Part model, mm, in its own coordinate system. Face numbers are marked on the shaded views. Round coordinates to 2 decimals unless told otherwise and drop trailing zeros. Write each loop counter-clockwise with the first axis right and the second up, starting at its lowest first coordinate (ties: lowest second). Pieces come first, ordered by that corner, then holes. Notation, with made-up numbers: M 69.25,71.25 L 89.25,71.25 A26 cw 89.25,95.25 Z; hole C 5.5,-18 d9. An arc over 180 degrees is marked long. Use one line per item in the form item = value. Start each with the question number.
Item 1: Mould opens along X. For the marked faces 1, 2 and 3 say: +X half, -X half, draft (parallel to the pull), parting line (faces both ways), or undercut.
Item 2: Cut at C-C, the plane x = 45. Give the cut face in (y, z), then the cut area to 3 significant figures.
Item 3: Probe L1, parallel to X at y = 12.25, z = 0; L2, parallel to Y at x = -36, z = 30.5; L3, parallel to X at y = 15.5, z = 0. List the from-to ranges inside material, lowest first.
Item 4: Cut at D-D, the plane y = 18.5. Give the cut face in (x, z), then the cut area to 3 significant figures.
Item 5: Flat gauge pins, fed straight in: pin 1 Ø6 at (y, z) = (11.5, -18.5) entering from -X; pin 2 Ø8 at (x, y) = (-5, 20.5) entering from -Z; pin 3 Ø1.5 at (x, y) = (32, 20) entering from +Z. Where does each tip first touch, or does it go through?
Item 6: Cut at A-A, the plane z = 0. Give the cut face in (x, y).
Item 7: Cut at B-B, the plane x = 0. Give the cut face in (y, z), then the cut area to 3 significant figures.
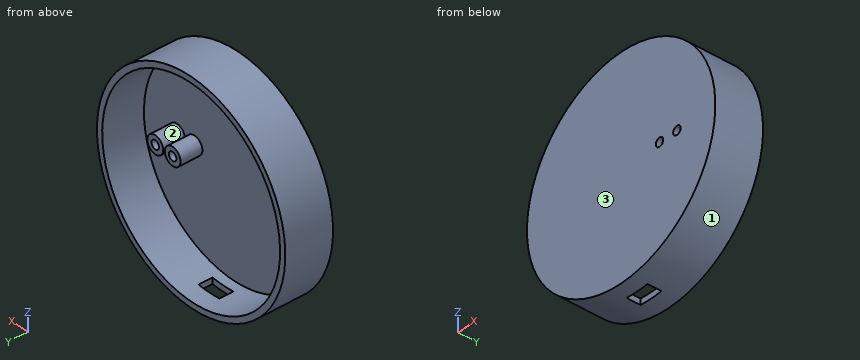
from build123d import *

# Parameters (mm, degrees)
SKETCH_1_R                     = 54
FLOOR_D108_T3_DEPTH            = 3
SKETCH_2_R                     = 54
SKETCH_2_R_2                   = 51
RIM_OD108_ID102_H24_DEPTH      = 24
SKETCH_3_R                     = 4.5
SENSOR_FIXED_POSTS_DEPTH       = 14
SKETCH_4_R                     = 2.15
M4_FIXED_MOUNT_CLEARANCE_DEPTH = 14
SKETCH_5_W                     = 12
SKETCH_5_H                     = 11
USB_C_SIDE_OPENING_12X7_DEPTH  = 7


with BuildPart() as part:
    # 草图1 → Floor_D108_T3 (new body)
    with BuildSketch(Plane(origin=(0, 0, 0), x_dir=(1, 0, 0), z_dir=(0, 1, 0))):
        with Locations(Location((0, 0, 0), (0, 0, 270))):
            Circle(SKETCH_1_R)
    extrude(amount=FLOOR_D108_T3_DEPTH)

    # 草图2 → Rim_OD108_ID102_H24 (add)
    with BuildSketch(Plane(origin=(0, 0, 0), x_dir=(1, 0, 0), z_dir=(0, 1, 0))):
        with Locations(Location((0, 0, 0), (0, 0, 270))):
            Circle(SKETCH_2_R)
        with Locations(Location((0, 0, 0), (0, 0, 270))):
            Circle(SKETCH_2_R_2, mode=Mode.SUBTRACT)
    extrude(amount=RIM_OD108_ID102_H24_DEPTH)

    # 草图3 → Sensor_fixed_posts (add)
    with BuildSketch(Plane(origin=(0, 0, 0), x_dir=(1, 0, 0), z_dir=(0, 1, 0))):
        with Locations(Location((22, 0, 0), (0, 0, 270))):
            Circle(SKETCH_3_R)
        with Locations(Location((32, 0, 0), (0, 0, 270))):
            Circle(SKETCH_3_R)
    extrude(amount=SENSOR_FIXED_POSTS_DEPTH)

    # 草图4 → M4_fixed_mount_clearance (cut)
    with BuildSketch(Plane(origin=(0, 0, 0), x_dir=(1, 0, 0), z_dir=(0, 1, 0))):
        with Locations(Location((22, 0, 0), (0, 0, 270))):
            Circle(SKETCH_4_R)
        with Locations(Location((32, 0, 0), (0, 0, 270))):
            Circle(SKETCH_4_R)
    extrude(amount=M4_FIXED_MOUNT_CLEARANCE_DEPTH, mode=Mode.SUBTRACT)

    # 草图5 → USB_C_side_opening_12x7 (cut)
    with BuildSketch(Plane(origin=(0, 8, 0), x_dir=(1, 0, 0), z_dir=(0, 1, 0))):
        with Locations((0, 54.5)):
            Rectangle(SKETCH_5_W, SKETCH_5_H)
    extrude(amount=USB_C_SIDE_OPENING_12X7_DEPTH, mode=Mode.SUBTRACT)


solid = part.part
Model answer:
q1.face_1 = parting line
q1.face_2 = undercut
q1.face_3 = draft
q2.outline = M 0,-29.85 L 24,-29.85 L 24,-24 L 3,-24 L 3,24 L 24,24 L 24,29.85 L 0,29.85 Z
q2.area = 425 mm²
q3.L1 = -54 to -51, 17.5 to 19.85, 24.15 to 26.5, 27.5 to 29.85, 34.15 to 36.5, 51 to 54
q3.L2 = 0 to 3
q3.L3 = -54 to -51, 51 to 54
q4.outline = C 0,0 d108; hole C 0,0 d102
q4.area = 990 mm²
q5.pin_1 = -51.73
q5.pin_2 = -53.99
q5.pin_3 = 44.04
q6.outline = M -54,0 L 19.85,0 L 19.85,14 L 17.5,14 L 17.5,3 L -51,3 L -51,24 L -54,24 Z; M 24.15,0 L 29.85,0 L 29.85,14 L 27.5,14 L 27.5,3 L 26.5,3 L 26.5,14 L 24.15,14 Z; M 34.15,0 L 54,0 L 54,24 L 51,24 L 51,3 L 36.5,3 L 36.5,14 L 34.15,14 Z
q7.outline = M 0,-54 L 8,-54 L 8,-51 L 3,-51 L 3,51 L 24,51 L 24,54 L 0,54 Z; M 15,-54 L 24,-54 L 24,-51 L 15,-51 Z
q7.area = 429 mm²
